Design review of the part shown in the three views and the two pictorial views. Dimensions are in mm from the part's minimum x, y and z. A direction names the side the tool comes from. Round coordinates to 2 decimals unless told otherwise and drop trailing zeros. Write each loop counter-clockwise with the first axis right and the second up, starting at its lowest first coordinate (ties: lowest second). Pieces come first, ordered by that corner, then holes. Notation, with made-up numbers: (61.5, 38.5) -> (91.5, 38.5) arc R34 ccw to (91.5, 75.5) -> close; hole circle Ø6 at (15, 31.5). An arc over 180 degrees is marked (long way). Answer as a JSON object with one key per item and string values. Group by question number.
1) We need section B-B, the plane x = 5.65. Write out the cut boundary in (y, z).
2) We need section C-C, the plane y = 11.5. Write out the cut boundary in (x, z).
3) We need section A-A, the plane y = 21.15. Write out the cut boundary in (x, z), then the cut area to 3 significant figures.
4) We need section D-D, the plane x = 17. Write out the cut boundary in (y, z).
5) To check wall thickness, follow probe 1 along Y at (x, z) = (36.65, 58.05); probe 2 along X at (y, z) = (36, 56); probe 3 along Z at (x, y) = (27, 25.5). State the ranges of each line that lie inside material, in increasing order. Write a range as [from, to].
6) Insertion check: pin 1 Ø1.5 at (x, y) = (6, 37) entering from +Z; pin 2 Ø1 at (x, y) = (16, 30) entering from +Z; pin 3 Ø4 at (x, y) = (36.65, 5.65) entering from +Z. Each pin has a flat end and moves straight along its axis. Give the tip position at first contact, or say it passes through.
7) Machinability: for the marked faces 1 and 2, which of the approach directions +Z, -Z, +X, -X, +Y, -Y give a long, thin tool a straight path to every point of the face, cutting with its end or side? Answer none if there is none.
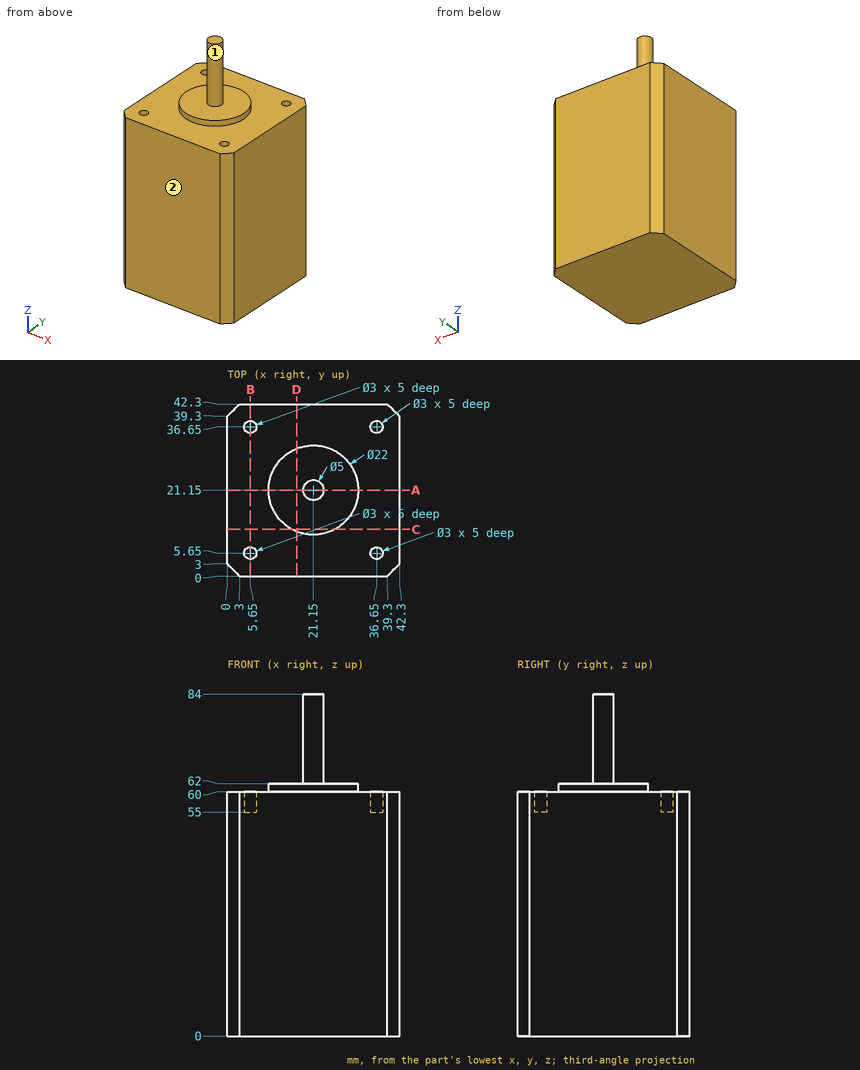
Here are the results:
{
 "1": {"outline": "(0, 0) -> (42.3, 0) -> (42.3, 60) -> (38.15, 60) -> (38.15, 55) -> (35.15, 55) -> (35.15, 60) -> (7.15, 60) -> (7.15, 55) -> (4.15, 55) -> (4.15, 60) -> (0, 60) -> close"},
 "2": {"outline": "(0, 0) -> (42.3, 0) -> (42.3, 60) -> (26.43, 60) -> (26.43, 62) -> (15.87, 62) -> (15.87, 60) -> (0, 60) -> close"},
 "3": {"outline": "(0, 0) -> (42.3, 0) -> (42.3, 60) -> (32.15, 60) -> (32.15, 62) -> (23.65, 62) -> (23.65, 84) -> (18.65, 84) -> (18.65, 62) -> (10.15, 62) -> (10.15, 60) -> (0, 60) -> close", "area": "2,690 mm^2"},
 "4": {"outline": "(0, 0) -> (42.3, 0) -> (42.3, 60) -> (31.34, 60) -> (31.34, 62) -> (10.96, 62) -> (10.96, 60) -> (0, 60) -> close"},
 "5": {"probe 1": "y = [0, 4.15], [7.15, 35.15], [38.15, 42.3]", "probe 2": "x = [0, 4.3], [7, 35.3], [38, 42.3]", "probe 3": "z = [0, 62]"},
 "6": {"pin 1": "stops at z = 55", "pin 2": "stops at z = 62", "pin 3": "stops at z = 60"},
 "7": {"face 1": "+Z", "face 2": "+Z, -Z, +X, -X, -Y"}
}
